Design review of the part built by this model. Coordinates are the model's own, in mm. Face numbers are marked on the shaded views. A direction names the side the tool comes from. Give positions to 0.01 mm unless a question says otherwise; leave off trailing zeros. Write each loop counter-clockwise with the first axis right and the second up, starting at its lowest first coordinate (ties: lowest second). Pieces come first, ordered by that corner, then holes. Notation, with made-up numbers: M -9,73.5 L 14,73.5 A16 cw 14,83.5 Z; hole C 2,-12.5 d1. An arc over 180 degrees is marked long. Use a Markdown table: item, result. Add a question column.
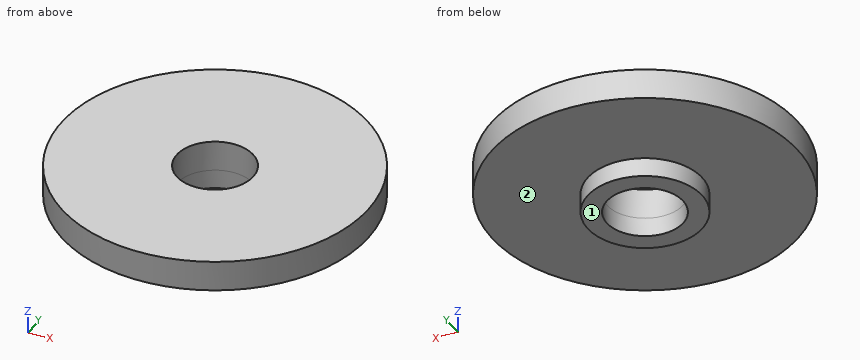
```python
from build123d import *

# Parameters (mm, degrees)
F0_R     = 40
F0_R_2   = 15
F0_R_3   = 10
F1_DEPTH = 8
F2_DEPTH = 5
F3_DEPTH = 5.001


with BuildPart() as f1:
    # F0 (on Top) → F1 (new body)
    with BuildSketch(Plane.XY):
        Circle(F0_R)
        Circle(F0_R_2, mode=Mode.SUBTRACT)
        Circle(F0_R_2)
        Circle(F0_R_3, mode=Mode.SUBTRACT)
    extrude(amount=F1_DEPTH)

    # F0 (on Top) → F2 (join)
    with BuildSketch(Plane.XY):
        Circle(F0_R_2)
        Circle(F0_R_3, mode=Mode.SUBTRACT)
    extrude(amount=-F2_DEPTH)

    # F0 (on Top) → F3 (cut, through all)
    with BuildSketch(Plane.XY):
        Circle(F0_R_3)
    extrude(amount=-F3_DEPTH, mode=Mode.SUBTRACT)


solid = f1.part
```
(1) Add section C-C on z = 5.75. Give the boundary of the cut face in (x, y), then the cut area to 3 significant figures.
(2) Wall thickness on L1, parallel to Y at x = 0, z = 2.25; L2, parallel to Y at x = 0, z = -3.95; L3, parallel to Z at x = -30, y = -20: over which ranges is each line inside the solid? List them lowest first.
(3) For pin 1 (12 mm diameter, centred on x = -18, y = 11.5, fed in from -Z), flat-tipped, find the tip position at first contact; note if it passes through.
(4) Add section A-A on x = 0. Give the boundary of the cut face in (y, z), then the cut area to 3 significant figures.
(5) Add section D-D on x = 14. Give the boundary of the cut face in (y, z), then the cut area to 3 significant figures.
(6) Machinability: for the marked faces 1 and 2, which of the approach directions +Z, -Z, +X, -X, +Y, -Y give a long, thin tool a straight path to every point of the face, cutting with its end or side? Answer none if there is none.
From the geometry:
| question | item | result |
|---|---|---|
| 1 | outline | C 0,0 d80; hole C 0,0 d20 |
| 1 | area | 4,710 mm^2 |
| 2 | L1 | y = -40 to -10, 10 to 40 |
| 2 | L2 | y = -15 to -10, 10 to 15 |
| 2 | L3 | z = 0 to 8 |
| 3 | pin 1 | stops at z = 0 |
| 4 | outline | M -40,0 L -15,0 L -15,-5 L -10,-5 L -10,8 L -40,8 Z; M 10,-5 L 15,-5 L 15,0 L 40,0 L 40,8 L 10,8 Z |
| 4 | area | 530 mm^2 |
| 5 | outline | M -37.47,0 L -5.39,0 L -5.39,-5 L 5.39,-5 L 5.39,0 L 37.47,0 L 37.47,8 L -37.47,8 Z |
| 5 | area | 653 mm^2 |
| 6 | face 1 | -Z, +X, -X, +Y, -Y |
| 6 | face 2 | -Z |
